Design review of the part built by this model. Coordinates are the model's own, in mm. A direction names the side the tool comes from. Round coordinates to 2 decimals unless told otherwise and drop trailing zeros. Order: outer loops, then holes, each group sorted by start corner. A loop starts at its lowest first (then second) coordinate and runs counter-clockwise, first axis right, second up. Notation, with made-up numbers: (8, 64.25) - (45, 64.25) arc R27 cw to (45, 101.25) - close; hole circle Ø4 at (37.5, 13.25). An arc over 180 degrees is marked (long way). Use CSV: the item, a comma, the result in double quotes.
Autodesk Fusion 360 part; units mm, degrees
sketch "Sketch1" plane through (0, 0, 0) normal (0, 0, 1) x (1, 0, 0)
  circle A0 centre (0, 0) radius 17.5
  circle A1 centre (0, 0) radius 12.5
  circle A2 centre (0, 0) radius 4.75
  dimension "d1" = 25
  dimension "d2" = 35
  dimension "d3" = 9.5
extrude "Extrude1" add sketch "Sketch1" along normal blind 4 contours A0 | A1
extrude "Extrude2" add sketch "Sketch1" against normal blind 110 contours A0
chamfer "Chamfer1" distance 5 angle 45 1 edges at (-16.3157, -6.3283, 4)
chamfer "Chamfer2" distance 2 angle 45 1 edges at (-11.6541, -4.5202, -110)
sketch "Sketch2" plane through (0, 0, 0) normal (0, 1, 0) x (1, 0, 0)
  line L0 (0, 108.9485) -> (-12.5, 108.9485)
  line L1 (0, 108.9485) -> (12.5, 108.9485)
  line L2 (-16, 108.9485) -> (-14, 108.9485)
  line L3 (-14, 108.9485) -> (-14, 104.4591)
  line L4 (-14, 104.4591) -> (-16, 104.4591)
  line L5 (-16, 104.4591) -> (-16, 108.9485)
  line L6 (14, 104.4591) -> (16, 104.4591)
  line L7 (16, 104.4591) -> (16, 108.9485)
  line L8 (16, 108.9485) -> (14, 108.9485)
  line L9 (14, 108.9485) -> (14, 104.4591)
  line L10 (-15, 118.4485) -> (-15, 99.4485)
  line L11 (15, 119.4485) -> (15, 98.4485)
  line L12 (-12.5, 108.9485) -> (-17.5, 108.9485)
  line L13 (12.5, 108.9485) -> (17.5, 108.9485)
  dimension "d10" = 12.5
  dimension "d11" = 12.5
  dimension "d12" = 2
  dimension "d13" = 2
  dimension "d14" = 5
  dimension "d15" = 5
extrude "Extrude3" cut sketch "Sketch2" along normal blind 100
extrude "Extrude4" cut 2 faces at (14.6667, 0, -107.452) (-15.3333, 0, -107.452) along direction (0, -1, 0) blind 100
chamfer "Chamfer3" distance 1 angle 45 4 edges at (14, 0, -104.4591) (-14, 0, -104.4591) (16, 0, -108.9485) (-16, 0, -108.9485)
equation "d10 = ( 25 / 2 ) * 1 mm"
1) To check wall thickness, follow L1, parallel to Y at x = 0, z = -33.5; L2, parallel to Z at x = -4, y = 8; L3, parallel to Y at x = 7.5, z = -71.5. State the ranges of each line that lie inside material, in increasing order. Write a range as from..to.
Data:
L1,"y = -17.5..-12.5, 12.5..17.5"
L2,"z = 0..4"
L3,"y = -15.81..-10, 10..15.81"
2) For faces 1 (the face through (-2.778, 12.508, 3.687)), 2 (the face through (-14, 0, -107)), 3 (the face through (11.923, 3.755, -53.244)), list the 3-axis set-ups (+Z, -Z, +X, -X, +Y, -Y) from which the entire face can be reached by the end or side of a thin tool; tool diameter is ignored.
Data:
face 1,"+Z"
face 2,"+Y, -Y"
face 3,"-Z"
3) We need section D-D (y = 6). Give the number of separate pieces and of enclosed holes in the cut face, then the cut area to 3 significant figures.
Data:
separate pieces,"1"
enclosed holes,"2"
area,"1,290 mm2"
4) We need section B-B (x = 0). Give the boundary of the cut face in (y, z).
Data:
outline,"(-17.5, -110) - (-14.5, -110) - (-12.5, -108) - (-12.5, 0) - (-4.75, 0) - (-4.75, 4) - (-12.5, 4) - (-17.5, -1) - close; (4.75, 0) - (12.5, 0) - (12.5, -108) - (14.5, -110) - (17.5, -110) - (17.5, -1) - (12.5, 4) - (4.75, 4) - close"
5) The part is to be moulded in two halves that separate along Y. For faces 4 (the face through (-2.737, 12.325, -108.125)), 5 (the face through (14, 0, -107)), 6 (the face through (-13.887, -10.648, -54.737)), say which applies: +Y half, -Y half, draft (parallel to the pull), parting line (faces both ways), or undercut.
Data:
face 4,"undercut"
face 5,"draft"
face 6,"parting line"
6) Insertion check: pin 1 Ø10 at (x, y) = (13.5, -12.5) entering from -Z; pin 2 Ø20 at (x, y) = (0, 0) entering from -Z; pin 3 Ø6 at (y, z) = (-12.5, -39.5) entering from -X; pin 4 Ø0.8 at (x, y) = (14.5, -5) entering from +Z. Each pin has a flat end and moves straight along its axis. Give the tip position at first contact, or say it passes through.
Data:
pin 1,"stops at z = -110"
pin 2,"stops at z = 0"
pin 3,"stops at x = -14.7"
pin 4,"stops at z = 1.56"
7) We need section A-A (y = 0). Give the boundary of the cut face in (x, z), then the cut area to 3 significant figures.
Data:
outline,"(-17.5, -110) - (-14.5, -110) - (-12.5, -108) - (-12.5, 0) - (-4.75, 0) - (-4.75, 4) - (-12.5, 4) - (-17.5, -1) - close; (4.75, 0) - (12.5, 0) - (12.5, -108) - (14.5, -110) - (17.5, -110) - (17.5, -1) - (12.5, 4) - (4.75, 4) - close; hole (-16, -107.95) - (-15, -108.95) - (-14, -108.95) - (-14, -105.46) - (-15, -104.46) - (-16, -104.46) - close; hole (14, -108.95) - (15, -108.95) - (16, -107.95) - (16, -104.46) - (15, -104.46) - (14, -105.46) - close"
area,"1,160 mm2"
8) We need section C-C (z = -72). Give the boundary of the cut face in (x, y).
Data:
outline,"circle Ø35 at (0, 0); hole circle Ø25 at (0, 0)"
